Input: part model. Units: mm. Frame: model coordinates. A direction names the side the tool comes from. Give positions to 0.01 mm unless a question says otherwise; leave off trailing zeros. Loops run counter-clockwise (first coordinate to the right, second up) from the corner with the lowest first, then second, coordinate; pieces in that order, holes last. Notation, with made-up numbers: (-5.5, -40) - (41.5, -40) arc R11 cw to (41.5, -26) - close; hole circle Ø3 at (75.25, 24.25). An arc over 180 degrees is marked (long way). One line per item, written item: value.
from build123d import *

# Parameters (mm, degrees)
F4_DEPTH  = 71.64283
F3_W      = 3.0015474185
F3_H      = 14.726341702
F5_DEPTH  = 20
F6_W      = 2.8139539063
F6_H      = 14.6325449459
F6_W_2    = 3.7519335747
F6_H_2    = 6.5658856183
F7_DEPTH  = 20
F9_DEPTH  = 20
F10_W     = 7.6914660167
F10_H     = 3.1891446561
F11_DEPTH = 20
F12_DEPTH = 49.92346


with BuildPart() as f1:
    # F0 (on Front) → F1 (revolve)
    with BuildSketch(Plane.XZ):
        Polygon((0, -24.5069297566), (0, 4.7725648619), (-4.554358311, 4.7725648619), (-19.2684326321, 4.7725648619), (-19.2684326321, -24.5069297566), align=None)
        Polygon((0, -43.7753610313), (0, -24.5069297566), (-19.2684326321, -24.5069297566), align=None)
    revolve(axis=Axis((0, 0, -9.8671824473), (0, 0, -1)))

    # F2 (on Top) → F4 (cut)
    with BuildSketch(Plane.XY):
        Polygon((-1.9789263333, -3.4276009537), (1.9789263333, -3.4276009537), (3.9578526666, 0), (1.9789263333, 3.4276009537), (-1.9789263333, 3.4276009537), (-3.9578526666, 0), align=None)
    extrude(amount=F4_DEPTH, mode=Mode.SUBTRACT)

    # F3 (on Right) → F5 (join)
    with BuildSketch(Plane.YZ):
        with Locations((6.941080559, -7.363170851)):
            Rectangle(F3_W, F3_H)
        Polygon((8.4418542683, -17.7278891206), (8.4418542683, -14.726341702), (5.4403068498, -14.726341702), (-6.9410782307, -14.726341702), (-6.9410782307, -17.7278891206), align=None)
    extrude(amount=F5_DEPTH)

    # F6 (on Right) → F7 (join)
    with BuildSketch(Plane.YZ):
        Polygon((9.0046431869, -3.2829423435), (9.0046431869, 0), (-8.4418542683, 0), (-8.4418542683, -3.2829423435), (-5.627900362, -3.2829423435), align=None)
        with Locations((-7.0348773152, -10.5992148165)):
            Rectangle(F6_W, F6_H)
        with Locations((6.5658842213, -14.6325444803)):
            Rectangle(F6_W_2, F6_H_2)
    extrude(amount=-F7_DEPTH)

    # F8 (on Front) → F9 (join)
    with BuildSketch(Plane.XZ):
        Polygon((8.4418524057, 0), (-6.7534814589, 0), (-6.7534814589, -3.8457328919), (4.1271289811, -3.8457328919), (8.4418524057, -3.8457328919), align=None)
        Polygon((8.4418524057, -18.4782778379), (8.4418524057, -3.8457328919), (4.1271289811, -3.8457328919), (4.1271289811, -6.0030948953), (4.1271289811, -11.1620053649), (4.1271289811, -18.4782778379), align=None)
        Polygon((4.1271289811, -11.1620053649), (4.1271289811, -6.0030948953), (0, -6.0030948953), (-7.1286750026, -18.1030835956), (-2.2027484971, -18.1030835956), (1.5007748734, -11.3496016711), align=None)
    extrude(amount=F9_DEPTH)

    # F10 (on Front) → F11 (join)
    with BuildSketch(Plane.XZ):
        Polygon((9.3798367307, -3.4705393482), (9.3798367307, 0), (-9.1922413558, 0), (-9.1922413558, -3.4705393482), (-6.1906939372, -3.4705393482), align=None)
        Polygon((-6.1906939372, -3.4705393482), (-9.1922413558, -3.4705393482), (-9.1922413558, -17.3526965082), (-6.1906939372, -17.3526965082), (-6.1906939372, -13.7883592397), align=None)
        Polygon((4.689917434, -13.7883592397), (-6.1906939372, -13.7883592397), (-6.1906939372, -17.3526965082), (9.0046431869, -17.3526965082), (9.0046431869, -13.7883592397), align=None)
        Polygon((4.689917434, -11.3496016711), (4.689917434, -13.7883592397), (9.0046431869, -13.7883592397), (9.0046431869, -8.160457015), (4.689917434, -8.160457015), align=None)
        with Locations((0.8441844257, -9.7550293431)):
            Rectangle(F10_W, F10_H)
    extrude(amount=-F11_DEPTH)

    # F2 (on Top) → F12 (cut)
    with BuildSketch(Plane.XY):
        Polygon((-1.9789263333, -3.4276009537), (1.9789263333, -3.4276009537), (3.9578526666, 0), (1.9789263333, 3.4276009537), (-1.9789263333, 3.4276009537), (-3.9578526666, 0), align=None)
    extrude(amount=-F12_DEPTH, mode=Mode.SUBTRACT)


solid = f1.part
Item 1: Section B-B, the plane z = -33.5. Output: boundary loops of the cut face in (x, y).
Verdict:
outline: circle Ø20.55 at (0, 0); hole (-3.96, 0) - (-1.98, -3.43) - (1.98, -3.43) - (3.96, 0) - (1.98, 3.43) - (-1.98, 3.43) - close
Item 2: Access query for faces 4 (the face through (9.005, 18, -13)), 5 (the face through (-19, -5.628, -11)), 6 (the face through (-5, -19, -18.103)). Directions: +Z, -Z, +X, -X, +Y, -Y. A direction counts if a zero-diameter tool reaches every point of the face in a straight line with its end or side. Return the directions, or none.
Verdict:
face 4: -Z, +X, +Y
face 5: -Z, -X
face 6: -Z, -X, -Y
Item 3: Material intervals for L1, parallel to X at y = -2, z = -28.5; L2, parallel to X at y = 3, z = -24; L3, parallel to X at y = 5.5, z = -7.5, sorted ascending.
Verdict:
L1: x = -15.14 to -2.8, 2.8 to 15.14
L2: x = -19.03 to -2.23, 2.23 to 19.03
L3: x = -18.47 to 20
Item 4: Pin query (flat end, axial travel): P1, Ø0.5, axis at x = -19.5, z = -12.5, coming from the +Y side; P2, Ø1, axis at x = -13.5, z = -15, coming from the +Y side; P3, Ø1, axis at x = 9, y = -1.5, coming from the -Z side. Return the tip coordinate at first contact, or that it passes through.
Verdict:
P1: stops at y = 8.44
P2: stops at y = 14.22
P3: stops at z = -35.15
Item 5: Section A-A, the plane z = -20.5. Output: boundary loops of the cut face in (x, y), and give its area (3 significant figures).
Verdict:
outline: circle Ø38.54 at (0, 0); hole (-3.96, 0) - (-1.98, -3.43) - (1.98, -3.43) - (3.96, 0) - (1.98, 3.43) - (-1.98, 3.43) - close
area: 1,130 mm^2
Item 6: Draft query along Z for faces 1 (the face through (-0.377, -19.565, -14.774)), 2 (the face through (3.2, 19.4, -3.471)), 3 (the face through (-2.955, 1.738, -18.103)). Return one class per face: pulls with the +Z half, pulls with the -Z half, needs draft (parallel to the pull), parting line crosses it, or undercut.
Verdict:
face 1: pulls with the -Z half
face 2: undercut
face 3: needs draft
